Geometry check sheet. Reference: the model listing, model coordinates, mm. A direction names the side the tool comes from. Give positions to 0.01 mm unless a question says otherwise; leave off trailing zeros. Loops run counter-clockwise (first coordinate to the right, second up) from the corner with the lowest first, then second, coordinate; pieces in that order, holes last. Notation, with made-up numbers: (6.25, 72.25) -> (38.25, 72.25) arc R29 ccw to (38.25, 105.25) -> close; hole circle Ø8 at (63, 60.25). An arc over 180 degrees is marked (long way). Write each question's results on one line, items separated by ' | '. Start each with the question number.
1) Sectioned sample at A-A on x = 0. Record the cut outline in (y, z).
2) Set-up check for faces 1 (the face through (-9.514, 1.014, -22.968)), 2 (the face through (1, 0, 10)): record each of +Z, -Z, +X, -X, +Y, -Y from which the full face is reachable in a straight line by a thin tool's end or side.
3) Sectioned sample at C-C on y = 0.7. Record the cut outline in (x, z), then the cut area to 3 significant figures.
4) Depth check by flat-ended pin: pin 1 (5 mm diameter, centred on x = -30.5, z = -34.5, fed in from -Y). Enter the tip coordinate at first touch or a pass-through.
5) Draft check along X on faces 3 (the face through (47.53, 1.01, -0.33)), 4 (the face through (1, 2, 10)), 5 (the face through (0, 1, -35)), 6 (the face through (15.02, 0.99, 47.69)). Enter one of: pulls with the +X half, pulls with the -X half, needs draft (parallel to the pull), parting line crosses it, or undercut.
6) Sectioned sample at D-D on x = -45. Record the cut outline in (y, z), then the cut area to 3 significant figures.
7) Scan lines: line 1 (X direction, y = 0.6, z = 0); line 2 (X direction, y = 1.5, z = 2); line 3 (Z direction, x = -45, y = 1.45). Record each from-to range of solid material in increasing order. Write a range as from..to.
8) Sectioned sample at B-B on z = 0. Record the cut outline in (x, y), then the cut area to 3 significant figures.
```python
from build123d import *

# Parameters (mm, degrees)
SKETCH2_R           = 50
BOSS_EXTRUDE1_DEPTH = 2
CUT_EXTRUDE1_REACH  = 72.739
SKETCH4_R           = 2.55
CUT_EXTRUDE2_DEPTH  = 71.738956735
CIRPATTERN1_COUNT   = 2
SKETCH5_R           = 1.5
CUT_EXTRUDE3_DEPTH  = 71.738956735


with BuildPart() as part:
    # Sketch2 → Boss-Extrude1 (new body)
    with BuildSketch(Plane(origin=(0, 0, 0), x_dir=(1, 0, 0), z_dir=(0, 1, 0))):
        with Locations(Location((0, 0, 0), (0, 0, 270))):
            Circle(SKETCH2_R)
    extrude(amount=BOSS_EXTRUDE1_DEPTH)

    # Sketch3 → Cut-Extrude1 (cut, up to next)
    with BuildSketch(Plane(origin=(0, 2, 0), x_dir=(1, 0, 0), z_dir=(0, 1, 0)), mode=Mode.PRIVATE) as cut_extrude1_sk1:
        with BuildLine():
            Line((-5.740251485, 13.858192988), (-13.393920133, 32.335783638))
            ThreePointArc((-13.393920133, 32.335783638), (0, 35), (13.393920133, 32.335783638))
            Line((13.393920133, 32.335783638), (5.740251485, 13.858192988))
            ThreePointArc((5.740251485, 13.858192988), (0, 15), (-5.740251485, 13.858192988))
        make_face()
    cut_extrude1_tool1 = extrude(cut_extrude1_sk1.sketch, amount=-CUT_EXTRUDE1_REACH, mode=Mode.PRIVATE) & part.part
    add(cut_extrude1_tool1.solids().sort_by_distance((0, 2, -25.661711))[0], mode=Mode.SUBTRACT)

    # Sketch4 → Cut-Extrude2 (cut, through all)
    with BuildSketch(Plane(origin=(0, 2, 0), x_dir=(1, 0, 0), z_dir=(0, 1, 0))):
        with Locations(Location((45, 0, 0), (0, 0, 270))):
            Circle(SKETCH4_R)
    cut_extrude2 = extrude(amount=-CUT_EXTRUDE2_DEPTH, mode=Mode.SUBTRACT)

    # CirPattern1: Cut-Extrude2 ×2 about axis
    cirpattern1_axis = Axis((0, 0, 0), (0, 1, 0))
    for i in range(1, CIRPATTERN1_COUNT):
        add(cut_extrude2.rotate(cirpattern1_axis, i * 360 / CIRPATTERN1_COUNT), mode=Mode.SUBTRACT)

    # Sketch5 → Cut-Extrude3 (cut, through all)
    with BuildSketch(Plane(origin=(0, 2, 0), x_dir=(1, 0, 0), z_dir=(0, 1, 0))):
        with Locations(Location((0, 0, 0), (0, 0, 270))):
            Circle(SKETCH5_R)
    extrude(amount=-CUT_EXTRUDE3_DEPTH, mode=Mode.SUBTRACT)


solid = part.part
```
Result:
1) outline: (0, -50) -> (2, -50) -> (2, -35) -> (0, -35) -> close; (0, -15) -> (2, -15) -> (2, -1.5) -> (0, -1.5) -> close; (0, 1.5) -> (2, 1.5) -> (2, 50) -> (0, 50) -> close
2) face 1: +Y, -Y | face 2: +Z, -Z, +X, -X, -Y
3) outline: circle Ø100 at (0, 0); hole circle Ø5.1 at (-45, 0); hole (-13.39, -32.34) arc R35 ccw to (13.39, -32.34) -> (5.74, -13.86) arc R15 cw to (-5.74, -13.86) -> close; hole circle Ø3 at (0, 0); hole circle Ø5.1 at (45, 0) | area: 7,410 mm^2
4) pin 1: y = 0
5) face 3: undercut | face 4: needs draft | face 5: undercut | face 6: parting line crosses it
6) outline: (0, -21.79) -> (2, -21.79) -> (2, -2.55) -> (0, -2.55) -> close; (0, 2.55) -> (2, 2.55) -> (2, 21.79) -> (0, 21.79) -> close | area: 77.0 mm^2
7) line 1: -50..-47.55, -42.45..-1.5, 1.5..42.45, 47.55..50 | line 2: -49.96..-46.58, -43.42..43.42, 46.58..49.96 | line 3: -21.79..-2.55, 2.55..21.79
8) outline: (-50, 0) -> (-47.55, 0) -> (-47.55, 2) -> (-50, 2) -> close; (-42.45, 0) -> (-1.5, 0) -> (-1.5, 2) -> (-42.45, 2) -> close; (1.5, 0) -> (42.45, 0) -> (42.45, 2) -> (1.5, 2) -> close; (47.55, 0) -> (50, 0) -> (50, 2) -> (47.55, 2) -> close | area: 174 mm^2
